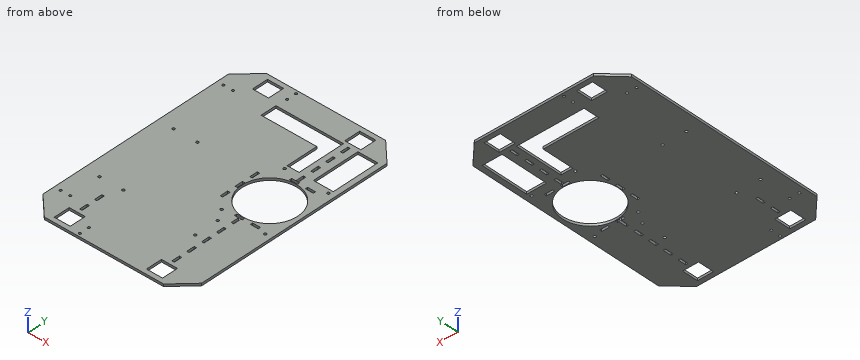
```python
from build123d import *

# Parameters (mm, degrees)
BASE_DEPTH                      = 3
ESQUISSE3_W                     = 20.2
ESQUISSE3_H                     = 20.2
ENL_V_MAT_EXTRU_1_DEPTH         = 4
R_P_TITION_LIN_AIRE1_COUNT      = 2
R_P_TITION_LIN_AIRE1_PITCH      = 267.5
R_P_TITION_LIN_AIRE1_COUNT_DIR2 = 2
R_P_TITION_LIN_AIRE1_PITCH_DIR2 = 116
ESQUISSE4_R                     = 35
ENL_V_MAT_EXTRU_2_DEPTH         = 4
ESQUISSE5_R                     = 1.625
ENL_V_MAT_EXTRU_3_DEPTH         = 3
R_P_TITION_LIN_AIRE2_COUNT      = 2
R_P_TITION_LIN_AIRE2_PITCH      = 85
R_P_TITION_LIN_AIRE2_COUNT_DIR2 = 2
R_P_TITION_LIN_AIRE2_PITCH_DIR2 = 55
ENL_V_MAT_EXTRU_4_REACH         = 5
ESQUISSE6_W                     = 25
ESQUISSE6_H                     = 60
ESQUISSE8_R                     = 1.5
TROUS_DEGUISEMENT_DEPTH         = 5
SKETCH1_W                       = 3
SKETCH1_H                       = 10
CUT_EXTRUDE1_DEPTH              = 4
LPATTERN1_COUNT                 = 5
LPATTERN1_PITCH                 = 20
SKETCH2_W                       = 3
SKETCH2_H                       = 10
CUT_EXTRUDE2_DEPTH              = 4
LPATTERN2_COUNT                 = 2
LPATTERN2_PITCH                 = 20
SKETCH3_W                       = 3
SKETCH3_H                       = 10
CUT_EXTRUDE3_DEPTH              = 4
LPATTERN3_COUNT                 = 4
LPATTERN3_PITCH                 = 20
ESQUISSE9_R                     = 1.625
ENL_V_MAT_EXTRU_5_DEPTH         = 10
ESQUISSE10_W                    = 10
ESQUISSE10_H                    = 3
ENL_V_MAT_EXTRU_6_DEPTH         = 3
ESQUISSE11_W                    = 3
ESQUISSE11_H                    = 10
ENL_V_MAT_EXTRU_7_DEPTH         = 3


with BuildPart() as part:
    # Esquisse1 → Base (new body)
    with BuildSketch(Plane.XY):
        Polygon((24.748737342, 24.748737342), (0, 0), (-150, 0), (-174.748737342, 24.748737342), (-174.748737342, 274.748737342), (-150, 299.497474683), (0, 299.497474683), (24.748737342, 274.748737342), align=None)
    extrude(amount=BASE_DEPTH)

    # Esquisse3 → Enlèv. mat.-Extru.1 (cut, through all)
    with BuildSketch(Plane.XY.offset(3)):
        with Locations((-132.998737342, 16)):
            Rectangle(ESQUISSE3_W, ESQUISSE3_H)
    enl_v_mat_extru_1 = extrude(amount=-ENL_V_MAT_EXTRU_1_DEPTH, mode=Mode.SUBTRACT)

    # Répétition linéaire1: Enl_v. mat.-Extru.1 2 × 2
    with Locations(*[(j * R_P_TITION_LIN_AIRE1_PITCH_DIR2, i * R_P_TITION_LIN_AIRE1_PITCH, 0) for i in range(R_P_TITION_LIN_AIRE1_COUNT) for j in range(R_P_TITION_LIN_AIRE1_COUNT_DIR2) if (i, j) != (0, 0)]):
        add(enl_v_mat_extru_1, mode=Mode.SUBTRACT)

    # Esquisse4 → Enlèv. mat.-Extru.2 (cut, through all)
    with BuildSketch(Plane.XY.offset(3)):
        with Locations((-15.251262658, 159.497474683)):
            Circle(ESQUISSE4_R)
    extrude(amount=-ENL_V_MAT_EXTRU_2_DEPTH, mode=Mode.SUBTRACT)

    # Esquisse5 → Enlèv. mat.-Extru.3 (cut)
    with BuildSketch(Plane.XY.offset(3)):
        with Locations((16.398737342, 119.65)):
            Circle(ESQUISSE5_R)
    enl_v_mat_extru_3 = extrude(amount=-ENL_V_MAT_EXTRU_3_DEPTH, mode=Mode.SUBTRACT)

    # Répétition linéaire2: Enl_v. mat.-Extru.3 2 × 2
    with Locations(*[(-j * R_P_TITION_LIN_AIRE2_PITCH_DIR2, i * R_P_TITION_LIN_AIRE2_PITCH, 0) for i in range(R_P_TITION_LIN_AIRE2_COUNT) for j in range(R_P_TITION_LIN_AIRE2_COUNT_DIR2) if (i, j) != (0, 0)]):
        add(enl_v_mat_extru_3, mode=Mode.SUBTRACT)

    # Esquisse6 → Enlèv. mat.-Extru.4 (cut, up to next)
    with BuildSketch(Plane.XY.offset(3), mode=Mode.PRIVATE) as enl_v_mat_extru_4_sk1:
        Polygon((-110, 269.497474683), (-40, 269.497474683), (-25, 269.497474683), (-25, 209.497474683), (-40, 209.497474683), (-40, 249.497474683), (-110, 249.497474683), align=None)
    enl_v_mat_extru_4_tool1 = extrude(enl_v_mat_extru_4_sk1.sketch, amount=-ENL_V_MAT_EXTRU_4_REACH, mode=Mode.PRIVATE) & part.part
    add(enl_v_mat_extru_4_tool1.solids().sort_by_distance((-58.369565, 251.671388, 3))[0], mode=Mode.SUBTRACT)
    # Esquisse6 → Enlèv. mat.-Extru.4 (cut, up to next)
    with BuildSketch(Plane.XY.offset(3), mode=Mode.PRIVATE) as enl_v_mat_extru_4_sk2:
        with Locations((5.601262658, 239.497474683)):
            Rectangle(ESQUISSE6_W, ESQUISSE6_H)
    enl_v_mat_extru_4_tool2 = extrude(enl_v_mat_extru_4_sk2.sketch, amount=-ENL_V_MAT_EXTRU_4_REACH, mode=Mode.PRIVATE) & part.part
    add(enl_v_mat_extru_4_tool2.solids().sort_by_distance((5.601263, 239.497475, 3))[0], mode=Mode.SUBTRACT)

    # Esquisse8 → Trous deguisement (cut)
    with BuildSketch(Plane.XY.offset(3)):
        with Locations((-109, 295.497474683)):
            Circle(ESQUISSE8_R)
        with Locations((-109, 283.497474683)):
            Circle(ESQUISSE8_R)
        with Locations((-166.748737342, 259.497474683)):
            Circle(ESQUISSE8_R)
        with Locations((-154.748737342, 259.497474683)):
            Circle(ESQUISSE8_R)
        with Locations((-109, 16)):
            Circle(ESQUISSE8_R)
        with Locations((-109, 4)):
            Circle(ESQUISSE8_R)
        with Locations((-154.748737342, 40)):
            Circle(ESQUISSE8_R)
        with Locations((-166.748737342, 40)):
            Circle(ESQUISSE8_R)
    extrude(amount=-TROUS_DEGUISEMENT_DEPTH, mode=Mode.SUBTRACT)

    # Sketch1 → Cut-Extrude1 (cut, through all)
    with BuildSketch(Plane.XY.offset(3)):
        with Locations((-16.998737342, 36.1)):
            Rectangle(SKETCH1_W, SKETCH1_H)
    cut_extrude1 = extrude(amount=-CUT_EXTRUDE1_DEPTH, mode=Mode.SUBTRACT)

    # LPattern1: Cut-Extrude1 ×5
    with Locations(*[(0, i * LPATTERN1_PITCH, 0) for i in range(1, LPATTERN1_COUNT)]):
        add(cut_extrude1, mode=Mode.SUBTRACT)

    # Sketch2 → Cut-Extrude2 (cut, through all)
    with BuildSketch(Plane.XY.offset(3)):
        with Locations((-132.998737342, 36.1)):
            Rectangle(SKETCH2_W, SKETCH2_H)
    cut_extrude2 = extrude(amount=-CUT_EXTRUDE2_DEPTH, mode=Mode.SUBTRACT)

    # LPattern2: Cut-Extrude2 ×2
    with Locations(*[(0, i * LPATTERN2_PITCH, 0) for i in range(1, LPATTERN2_COUNT)]):
        add(cut_extrude2, mode=Mode.SUBTRACT)

    # Sketch3 → Cut-Extrude3 (cut, through all)
    with BuildSketch(Plane.XY.offset(3)):
        with Locations((-16.998737342, 263.4)):
            Rectangle(SKETCH3_W, SKETCH3_H)
    cut_extrude3 = extrude(amount=-CUT_EXTRUDE3_DEPTH, mode=Mode.SUBTRACT)

    # LPattern3: Cut-Extrude3 ×4
    with Locations(*[(0, -i * LPATTERN3_PITCH, 0) for i in range(1, LPATTERN3_COUNT)]):
        add(cut_extrude3, mode=Mode.SUBTRACT)

    # Esquisse9 → Enlèv. mat.-Extru.5 (cut)
    with BuildSketch(Plane.XY.offset(3)):
        with Locations((-154.748737342, 179.497474683)):
            Circle(ESQUISSE9_R)
        with Locations((-124.748737342, 179.497474683)):
            Circle(ESQUISSE9_R)
        with Locations((-154.748737342, 79.497474683)):
            Circle(ESQUISSE9_R)
        with Locations((-124.748737342, 79.497474683)):
            Circle(ESQUISSE9_R)
        with Locations((-29.748737342, 74.65)):
            Circle(ESQUISSE9_R)
        with Locations((-29.748737342, 104.65)):
            Circle(ESQUISSE9_R)
    extrude(amount=-ENL_V_MAT_EXTRU_5_DEPTH, mode=Mode.SUBTRACT)

    # Esquisse10 → Enlèv. mat.-Extru.6 (cut)
    with BuildSketch(Plane.XY.offset(3)):
        with Locations((1.298737342, 122.4)):
            Rectangle(ESQUISSE10_W, ESQUISSE10_H)
        with Locations((-18.701262658, 122.4)):
            Rectangle(ESQUISSE10_W, ESQUISSE10_H)
        with Locations((-18.701262658, 196.697474683)):
            Rectangle(ESQUISSE10_W, ESQUISSE10_H)
        with Locations((1.298737342, 196.697474683)):
            Rectangle(ESQUISSE10_W, ESQUISSE10_H)
    extrude(amount=-ENL_V_MAT_EXTRU_6_DEPTH, mode=Mode.SUBTRACT)

    # Esquisse11 → Enlèv. mat.-Extru.7 (cut)
    with BuildSketch(Plane.XY.offset(3)):
        with Locations((-52.201262658, 158.9)):
            Rectangle(ESQUISSE11_W, ESQUISSE11_H)
        with Locations((-52.201262658, 138.9)):
            Rectangle(ESQUISSE11_W, ESQUISSE11_H)
        with Locations((-52.201262658, 178.9)):
            Rectangle(ESQUISSE11_W, ESQUISSE11_H)
    extrude(amount=-ENL_V_MAT_EXTRU_7_DEPTH, mode=Mode.SUBTRACT)


solid = part.part
```
Here's how the part is built. I have some questions about the finished solid (model axes, mm). Coordinates: 2 decimals unless noted, no trailing zeros. Loops run counter-clockwise (first coordinate to the right, second up) from the corner with the lowest first, then second, coordinate; pieces in that order, holes last. Notation, with made-up numbers: (72.5, 56.25) - (131.5, 56.25) arc R25 cw to (131.5, 79.25) - close; hole circle Ø6 at (-5.75, 76). An arc over 180 degrees is marked (long way). Return JSON: item names as keys, results as strings. Group by question number.
Item 1: If we section it at D-D on z = 1.6: State how many separate pieces and enclosed holes the cut face has, and give its area (3 significant figures).
Item 2: Will these pins go through, and if not, where does the flat tip stop? P1, Ø1.5, axis at x = 3, z = 1.5, coming from the -Y side; P2, Ø4, axis at x = -34.5, y = 210.5, coming from the +Z side; P3, Ø0.9, axis at y = 11.5, z = 1, coming from the +X side.
Item 3: If we section it at C-C on x = -162: Write out the boundary of the cut face in (y, z), and give its area (3 significant figures).
Item 4: I need wall thicknesses on line 1 (Y direction, x = -53, z = 2.35); line 2 (Y direction, x = -134, z = 1.65); line 3 (X direction, y = 252.5, z = 1.4). Which ranges of each line are inside material? Lowest first, please. Write a range as from..to.
Item 5: If we section it at B-B on x = -79: Write out the boundary of the cut face in (y, z).
Item 6: If we section it at A-A on y = 215.5: Write out the boundary of the cut face in (x, z).
Calculated:
{
 "1": {"separate pieces": "1", "enclosed holes": "42", "area": "48,600 mm^2"},
 "2": {"P1": "stops at y = 2.25", "P2": "stops at z = 3", "P3": "stops at x = 11.95"},
 "3": {"outline": "(12, 0) - (287.5, 0) - (287.5, 3) - (12, 3) - close", "area": "826 mm^2"},
 "4": {"line 1": "y = 0..133.9, 143.9..153.9, 163.9..173.9, 183.9..249.5, 269.5..299.5", "line 2": "y = 0..5.9, 26.1..31.1, 41.1..51.1, 61.1..273.4, 293.6..299.5", "line 3": "x = -174.75..-110, -25..-6.9, 18.1..24.75"},
 "5": {"outline": "(0, 0) - (249.5, 0) - (249.5, 3) - (0, 3) - close; (269.5, 0) - (299.5, 0) - (299.5, 3) - (269.5, 3) - close"},
 "6": {"outline": "(-174.75, 0) - (-40, 0) - (-40, 3) - (-174.75, 3) - close; (-25, 0) - (-6.9, 0) - (-6.9, 3) - (-25, 3) - close; (18.1, 0) - (24.75, 0) - (24.75, 3) - (18.1, 3) - close"}
}
